from build123d import *

# Parameters (mm, degrees)
CYLINDER056_R     = 3.15
CYLINDER056_DEPTH = 10
CYLINDER055_R     = 3.15
CYLINDER055_DEPTH = 10
CYLINDER_R        = 3.15
CYLINDER_DEPTH    = 10
CYLINDER057_R     = 3.15
CYLINDER057_DEPTH = 10
BOX002_W          = 5
BOX002_H          = 5
BOX002_DEPTH      = 5
BOX001_W          = 59.5
BOX001_H          = 27
BOX001_DEPTH      = 5
BOX_W             = 86.5
BOX_H             = 44
BOX_DEPTH         = 5
CHAMFER_SIZE      = 4
FILLET_R          = 3
FILLET001_R       = 1


with BuildPart() as cylinder056:
    # Cylinder056 → Cylinder056 (new body)
    with BuildSketch(Plane(origin=(-15, -34, 26.5), x_dir=(1, 0, 0), z_dir=(0, 0, 1))):
        Circle(CYLINDER056_R)
    extrude(amount=CYLINDER056_DEPTH)


with BuildPart() as cylinder055:
    # Cylinder055 → Cylinder055 (new body)
    with BuildSketch(Plane(origin=(10, 15, 26.5), x_dir=(1, 0, 0), z_dir=(0, 0, 1))):
        Circle(CYLINDER055_R)
    extrude(amount=CYLINDER055_DEPTH)


with BuildPart() as cylinder:
    # Cylinder → Cylinder (new body)
    with BuildSketch(Plane(origin=(-15, -10, 26.5), x_dir=(1, 0, 0), z_dir=(0, 0, 1))):
        Circle(CYLINDER_R)
    extrude(amount=CYLINDER_DEPTH)


with BuildPart() as fusion006002011004053036004001002:
    # Cylinder057 → Cylinder057 (new body)
    with BuildSketch(Plane(origin=(49.5, 15, 26.5), x_dir=(1, 0, 0), z_dir=(0, 0, 1))):
        Circle(CYLINDER057_R)
    extrude(amount=CYLINDER057_DEPTH)

    # Fusion006002011004053036004001002: union Cylinder056, Cylinder055, Cylinder
    add(cylinder056.part)
    add(cylinder055.part)
    add(cylinder.part)


with BuildPart() as cube002:
    # Box002 → Box002 (new body)
    with BuildSketch(Plane(origin=(-1, -4, 30), x_dir=(1, 0, 0), z_dir=(0, 0, 1))):
        with Locations((2.5, 2.5)):
            Rectangle(BOX002_W, BOX002_H)
    extrude(amount=BOX002_DEPTH)


with BuildPart() as cube001:
    # Box001 → Box001 (new body)
    with BuildSketch(Plane.XY.offset(30)):
        with Locations((29.75, 13.5)):
            Rectangle(BOX001_W, BOX001_H)
    extrude(amount=BOX001_DEPTH)


with BuildPart() as base_plate:
    # Box → Box (new body)
    with BuildSketch(Plane(origin=(-27, -44, 30), x_dir=(1, 0, 0), z_dir=(0, 0, 1))):
        with Locations((43.25, 22)):
            Rectangle(BOX_W, BOX_H)
    extrude(amount=BOX_DEPTH)

    # Fusion: union Cube001
    add(cube001.part)

    # Cut: cut Cube002
    add(cube002.part, mode=Mode.SUBTRACT)

    # Chamfer
    chamfer_edges = [base_plate.edges().sort_by_distance(p)[0] for p in [
        (59.5, -44, 32.5),
    ]]
    chamfer(chamfer_edges, length=CHAMFER_SIZE)

    # Fillet
    fillet_edges = [base_plate.edges().sort_by_distance(p)[0] for p in [
        (-27, -44, 32.5),
        (-27, 0, 32.5),
        (59.5, 27, 32.5),
        (0, 27, 32.5),
    ]]
    fillet(fillet_edges, radius=FILLET_R)

    # Fillet001
    fillet001_edges = [base_plate.edges().sort_by_distance(p)[0] for p in [
        (-1, 0, 32.5),
        (4, -4, 32.5),
        (4, 1, 32.5),
        (-1, -4, 32.5),
        (0, 1, 32.5),
    ]]
    fillet(fillet001_edges, radius=FILLET001_R)

    # Cut002008: cut Fusion006002011004053036004001002
    add(fusion006002011004053036004001002.part, mode=Mode.SUBTRACT)


solid = base_plate.part
Work out the finished part from the listing and answer in its coordinate system (mm). A direction names the side the tool comes from. Coordinates: 2 decimals unless noted, no trailing zeros. Write each loop counter-clockwise with the first axis right and the second up, starting at its lowest first coordinate (ties: lowest second). Pieces come first, ordered by that corner, then holes. Notation, with made-up numbers: M 79.5,27 L 83.5,27 A18 ccw 83.5,38 Z; hole C 6,51.5 d11. An arc over 180 degrees is marked long. Write item = value, one per line.
1. The part is cut by section D-D (x = -15). Determine the outline of the cut face in (y, z), then the cut area to 3 significant figures.
Solution:
outline = M -44,30 L -37.15,30 L -37.15,35 L -44,35 Z; M -30.85,30 L -13.15,30 L -13.15,35 L -30.85,35 Z; M -6.85,30 L 0,30 L 0,35 L -6.85,35 Z
area = 157 mm2
2. Straight lines are drawn through the part: line 1 (X direction, y = 15, z = 33.7); line 2 (Y direction, x = -15, z = 31.75); line 3 (Y direction, x = 49.5, z = 33.55). For each, find the intervals that lie inside material, in ascending order. Write a range as from..to.
Solution:
line_1 = 0..6.85, 13.15..46.35, 52.65..59.5
line_2 = -44..-37.15, -30.85..-13.15, -6.85..0
line_3 = -44..11.85, 18.15..27
3. The part is cut by section B-B (z = 33.15). Determine the outline of the cut face in (x, y), then the cut area to 3 significant figures.
Solution:
outline = M -27,-41 A3 ccw -24,-44 L 55.5,-44 L 59.5,-40 L 59.5,24 A3 ccw 56.5,27 L 3,27 A3 ccw 0,24 L 0,2 A1 ccw 1,1 L 3,1 A1 cw 4,0 L 4,-3 A1 cw 3,-4 L 0,-4 A1 cw -1,-3 L -1,-1 A1 ccw -2,0 L -24,0 A3 ccw -27,-3 Z; hole C -15,-34 d6.3; hole C -15,-10 d6.3; hole C 10,15 d6.3; hole C 49.5,15 d6.3
area = 5,250 mm2
4. The part is cut by section A-A (y = 15). Determine the outline of the cut face in (x, z), then the cut area to 4 significant figures.
Solution:
outline = M 0,30 L 6.85,30 L 6.85,35 L 0,35 Z; M 13.15,30 L 46.35,30 L 46.35,35 L 13.15,35 Z; M 52.65,30 L 59.5,30 L 59.5,35 L 52.65,35 Z
area = 234.5 mm2
5. The part is cut by section C-C (x = 49.5). Determine the outline of the cut face in (y, z).
Solution:
outline = M -44,30 L 11.85,30 L 11.85,35 L -44,35 Z; M 18.15,30 L 27,30 L 27,35 L 18.15,35 Z
6. Determine the mould class of faces 6 (the face through (-13, 0, 32)), 7 (the face through (-27, -22, 32)), 8 (the face through (-17.32, -7.87, 32.47)), 9 (the face through (7.5, 13.083, 32.465)) for opening direction Y: released by +Y, released by -Y, zero draft, split by the parting line, or undercut.
Solution:
face_6 = released by +Y
face_7 = zero draft
face_8 = undercut
face_9 = undercut
7. For faces 1 (the face through (2, 1, 32)), 2 (the face through (-1, -2, 32)), 3 (the face through (16, -8, 35)), 4 (the face through (1, -4, 32)), 5 (the face through (0, 13, 32)), determine the directions among +Z, -Z, +X, -X, +Y, -Y from which every point of the face is accessible in a straight line to the end or side of a thin tool.
Solution:
face_1 = +Z, -Z, -X
face_2 = +Z, -Z, +Y
face_3 = +Z, +X, -X, +Y, -Y
face_4 = +Z, -Z
face_5 = +Z, -Z, -X, +Y
8. A flat-ended cylindrical pin translates along its axis: pin 1 (2.5 mm diameter, centred on y = 14, z = 33.5, fed in from -X). Find the tip coordinate at first contact, or state that the pin passes through.
Solution:
pin_1 = 0
